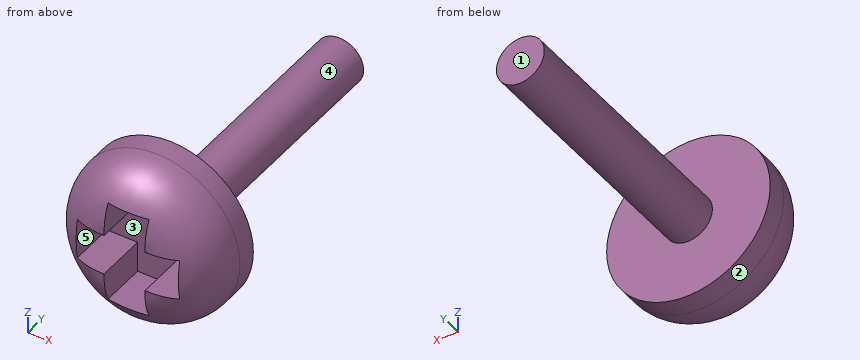
```python
from build123d import *

# Parameters (mm, degrees)
SKETCH1_R           = 0.5953125
BOSS_EXTRUDE1_DEPTH = 3.175
SKETCH2_R           = 2.032
BOSS_EXTRUDE2_DEPTH = 1.778
FILLET1_R           = 1.27
CUT_EXTRUDE1_DEPTH  = 1.27


with BuildPart() as part:
    # Sketch1 → Boss-Extrude1 (new body, symmetric)
    with BuildSketch(Plane(origin=(0, 0, 0), x_dir=(1, 0, 0), z_dir=(0, 1, 0))):
        Circle(SKETCH1_R)
    extrude(amount=BOSS_EXTRUDE1_DEPTH, both=True)

    # Sketch2 → Boss-Extrude2 (add)
    with BuildSketch(Plane.XZ.offset(3.175)):
        Circle(SKETCH2_R)
    extrude(amount=BOSS_EXTRUDE2_DEPTH)

    # Fillet1
    fillet1_edges = [part.edges().sort_by_distance(p)[0] for p in [
        (-2.032, -4.953, 0),
    ]]
    fillet(fillet1_edges, radius=FILLET1_R)

    # Sketch3 → Cut-Extrude1 (cut)
    with BuildSketch(Plane.XZ.offset(4.953)):
        Polygon((-0.508, -0.508), (-1.27, -0.508), (-1.27, 0.508), (-0.508, 0.508), (-0.508, 1.27), (0.508, 1.27), (0.508, 0.508), (1.27, 0.508), (1.27, -0.508), (0.508, -0.508), (0.508, -1.27), (-0.508, -1.27), align=None)
    extrude(amount=-CUT_EXTRUDE1_DEPTH, mode=Mode.SUBTRACT)


solid = part.part
```
Source: CAD feature listing. Evaluate the final solid. Frame: model axes, mm. Face numbers are marked on the shaded views. A direction names the side the tool comes from. Give positions to 0.01 mm unless a question says otherwise; leave off trailing zeros. Order: outer loops, then holes, each group sorted by start corner. A loop starts at its lowest first (then second) coordinate and runs counter-clockwise, first axis right, second up.
(1) Contact query for flat-ended pins moving along their axis: P1, Ø0.8, axis at x = -1, y = -4.5, coming from the -Z side; P2, Ø0.8, axis at y = -4.5, z = -1, coming from the +X side; P3, Ø1.5, axis at y = -2, z = 0, coming from the +X side. Output: stop coordinate, or through.
(2) Pull-direction query (Z, two-part tool) for the marked faces 1, 2 and 3; classes: +Z half, -Z half, draft (parallel to the pull), parting line (faces both ways), or undercut.
(3) Section query A-A (y = -1.25). Return the cut outline in (x, z).
(4) Access query for the marked faces 4 and 5. Directions: +Z, -Z, +X, -X, +Y, -Y. A direction counts if a zero-diameter tool reaches every point of the face in a straight line with its end or side. Return the directions, or none.
(5) Material intervals for line 1 along Y through (x, z) = (0.55, -0.4) (3 decimals); line 2 along Z through (x, y) = (0, 2.5); line 3 along Y through (x, z) = (-0.5, -0.2) (3 decimals), sorted ascending.
Outcome:
1. P1: stops at z = -1.78
1. P2: stops at x = 1.78
1. P3: stops at x = 0.6
2. face 1: draft
2. face 2: parting line
2. face 3: undercut
3. outline: circle Ø1.19 at (0, 0)
4. face 4: +Y
4. face 5: -Y
5. line 1: y = -3.683 to -3.175
5. line 2: z = -0.6 to 0.6
5. line 3: y = -3.683 to 3.175
